```python
from build123d import *

# Parameters (mm, degrees)
SKETCH1_W           = 22.6
SKETCH1_H           = 28.65
SKETCH1_W_2         = 12.6
SKETCH1_H_2         = 19.5
BOSS_EXTRUDE1_DEPTH = 14
SKETCH3_W           = 22.6
SKETCH3_H           = 7
BOSS_EXTRUDE2_DEPTH = 4
SKETCH4_W           = 22.6
SKETCH4_H           = 2
BOSS_EXTRUDE3_DEPTH = 10
SKETCH5_W           = 25.687080714
SKETCH5_H           = 15.752193048
CUT_EXTRUDE1_DEPTH  = 28.577164466


with BuildPart() as part:
    # Sketch1 → Boss-Extrude1 (new body)
    with BuildSketch(Plane.XY):
        with Locations((0, -0.425)):
            Rectangle(SKETCH1_W, SKETCH1_H)
        Rectangle(SKETCH1_W_2, SKETCH1_H_2, mode=Mode.SUBTRACT)
    extrude(amount=BOSS_EXTRUDE1_DEPTH)

    # Sketch3 → Boss-Extrude2 (add)
    with BuildSketch(Plane.XY.offset(10)):
        with Locations((0, 17.4)):
            Rectangle(SKETCH3_W, SKETCH3_H)
    extrude(amount=BOSS_EXTRUDE2_DEPTH)

    # Sketch4 → Boss-Extrude3 (add)
    with BuildSketch(Plane(origin=(0, 0, 10), x_dir=(-1, 0, 0), z_dir=(0, 0, -1))):
        with Locations((0, 19.9)):
            Rectangle(SKETCH4_W, SKETCH4_H)
    extrude(amount=BOSS_EXTRUDE3_DEPTH)

    # Sketch5 → Cut-Extrude1 (cut, through all)
    with BuildSketch(Plane.XY.offset(14)):
        with Locations((16.840510888, 23.946149684)):
            Rectangle(SKETCH5_W, SKETCH5_H)
    extrude(amount=-CUT_EXTRUDE1_DEPTH, mode=Mode.SUBTRACT)


solid = part.part
```
CAD build for the part. Positions are in the model's coordinates, mm. A direction names the side the tool comes from. Give positions to 0.01 mm unless a question says otherwise; leave off trailing zeros. Write each loop counter-clockwise with the first axis right and the second up, starting at its lowest first coordinate (ties: lowest second). Pieces come first, ordered by that corner, then holes. Notation, with made-up numbers: M 79.25,-27.5 L 107.25,-27.5 A17 ccw 107.25,3.5 Z; hole C 73,-25 d1. An arc over 180 degrees is marked long. Return JSON: item names as keys, results as strings. Group by question number.
(1) Band-saw the part on A-A (z = 7.75). Give the cut face in (x, y), and give its area (3 significant figures).
(2) Band-saw the part on C-C (y = -8). Give the cut face in (x, z).
(3) Mould opens along Y. For faces 1 (the face through (0, -9.75, 7)), 2 (the face through (0, -14.75, 7)), 3 (the face through (-3, 16, 10)), 4 (the face through (-4, 20.9, 7)) say: pulls with the +Y half, pulls with the -Y half, needs draft (parallel to the pull), parting line crosses it, or undercut.
(4) Flat gauge pins, fed straight in: pin 1 Ø4 at (x, y) = (-3, -7) entering from +Z; pin 2 Ø1 at (x, y) = (-5, 14.5) entering from -Z; pin 3 Ø3 at (x, z) = (7, 11.5) entering from +Y; pin 4 Ø5 at (x, y) = (4.5, 6.5) entering from -Z. Where does each tip first touch, or does it go through?
(5) Band-saw the part on D-D (x = -8). Give the cut face in (y, z).
(6) Band-saw the part on B-B (x = 3.5). Give the cut face in (y, z).
(7) Drill centre lines: L1, parallel to Y at x = -3.5, z = 7.25; L2, parallel to X at y = -1, z = 9.75; L3, parallel to Y at x = 6.25, z = 4. Where is each one in solid material? Low to high. Write a range as [from, to].
(8) 3-axis set-ups, long thin cutter, end or side, ignore diameter. For faces 5 (the face through (8, 16.07, 12)), 6 (the face through (0, 9.75, 7)), 7 (the face through (0, 13.9, 5)): which of +Z, -Z, +X, -X, +Y, -Y reach the whole face in a straight line?
Entries:
{
 "1": {"outline": "M -11.3,-14.75 L 11.3,-14.75 L 11.3,13.9 L -11.3,13.9 Z; M -11.3,18.9 L 4,18.9 L 4,20.9 L -11.3,20.9 Z; hole M -6.3,-9.75 L 6.3,-9.75 L 6.3,9.75 L -6.3,9.75 Z", "area": "432 mm^2"},
 "2": {"outline": "M -11.3,0 L -6.3,0 L -6.3,14 L -11.3,14 Z; M 6.3,0 L 11.3,0 L 11.3,14 L 6.3,14 Z"},
 "3": {"face 1": "undercut", "face 2": "pulls with the -Y half", "face 3": "undercut", "face 4": "pulls with the +Y half"},
 "4": {"pin 1": "passes through", "pin 2": "stops at z = 10", "pin 3": "stops at y = 16.07", "pin 4": "stops at z = 0"},
 "5": {"outline": "M -14.75,0 L 13.9,0 L 13.9,10 L 18.9,10 L 18.9,0 L 20.9,0 L 20.9,14 L -14.75,14 Z"},
 "6": {"outline": "M -14.75,0 L -9.75,0 L -9.75,14 L -14.75,14 Z; M 9.75,0 L 13.9,0 L 13.9,10 L 18.9,10 L 18.9,0 L 20.9,0 L 20.9,14 L 9.75,14 Z"},
 "7": {"L1": "y = [-14.75, -9.75], [9.75, 13.9], [18.9, 20.9]", "L2": "x = [-11.3, -6.3], [6.3, 11.3]", "L3": "y = [-14.75, -9.75], [9.75, 13.9]"},
 "8": {"face 5": "+Z, -Z, +X, +Y", "face 6": "+Z, -Z", "face 7": "-Z, +X, -X"}
}
